Verification items for the finished model (mm, model axes). Round coordinates to 2 decimals unless told otherwise and drop trailing zeros. Write each loop counter-clockwise with the first axis right and the second up, starting at its lowest first coordinate (ties: lowest second). Pieces come first, ordered by that corner, then holes. Notation, with made-up numbers: (20, -34.75) - (54, -34.75) arc R19 ccw to (54, -5.75) - close; hole circle Ø5 at (-10, -2). An arc over 180 degrees is marked (long way). Answer as a JSON object with one key per item and string values.
```python
from build123d import *

# Parameters (mm, degrees)
SKETCH1_W           = 120
SKETCH1_H           = 50
BOSS_EXTRUDE1_DEPTH = 5
SKETCH4_R           = 17.4
CUT_EXTRUDE3_DEPTH  = 2
CUT_EXTRUDE2_DEPTH  = 5
BOSS_EXTRUDE2_DEPTH = 4
CIRPATTERN1_COUNT   = 4
SKETCH6_R           = 1.6
CUT_EXTRUDE4_DEPTH  = 131.096118313
SKETCH8_W           = 56
SKETCH8_H           = 28
CUT_EXTRUDE5_DEPTH  = 131.096118313
SKETCH9_W           = 44
SKETCH9_H           = 40
CUT_EXTRUDE6_DEPTH  = 3
SKETCH10_W          = 56
SKETCH10_H          = 40
CUT_EXTRUDE7_DEPTH  = 1
SKETCH11_R          = 1.6
CUT_EXTRUDE8_DEPTH  = 131.096118313
CHAMFER1_SIZE       = 1
CHAMFER2_SIZE       = 1


with BuildPart() as part:
    # Sketch1 → Boss-Extrude1 (new body)
    with BuildSketch(Plane(origin=(0, 0, 0), x_dir=(1, 0, 0), z_dir=(0, 1, 0))):
        with Locations((60, 25)):
            Rectangle(SKETCH1_W, SKETCH1_H)
    extrude(amount=BOSS_EXTRUDE1_DEPTH)

    # Sketch4 → Cut-Extrude3 (cut)
    with BuildSketch(Plane(origin=(0, 5, 0), x_dir=(1, 0, 0), z_dir=(0, 1, 0))):
        with Locations(Location((25, 25, 0), (0, 0, 270))):
            Circle(SKETCH4_R)
    extrude(amount=-CUT_EXTRUDE3_DEPTH, mode=Mode.SUBTRACT)

    # Sketch3 → Cut-Extrude2 (cut)
    with BuildSketch(Plane(origin=(0, 5, 0), x_dir=(1, 0, 0), z_dir=(0, 1, 0))):
        with BuildLine():
            Line((15, 36.5), (35, 36.5))
            ThreePointArc((35, 36.5), (36.414213562, 35.914213562), (37, 34.5))
            Line((37, 34.5), (37, 15.5))
            ThreePointArc((37, 15.5), (36.414213562, 14.085786438), (35, 13.5))
            Line((35, 13.5), (15, 13.5))
            ThreePointArc((15, 13.5), (13.585786438, 14.085786438), (13, 15.5))
            Line((13, 15.5), (13, 34.5))
            ThreePointArc((13, 34.5), (13.585786438, 35.914213562), (15, 36.5))
        make_face()
    extrude(amount=-CUT_EXTRUDE2_DEPTH, mode=Mode.SUBTRACT)

    # Sketch5 → Boss-Extrude2 (add)
    with BuildSketch(Plane(origin=(0, 3, 0), x_dir=(1, 0, 0), z_dir=(0, 1, 0))):
        with BuildLine():
            Line((9.8, 28.75), (11, 28.75))
            ThreePointArc((11, 28.75), (11.282842712, 28.632842712), (11.4, 28.35))
            Line((11.4, 28.35), (11.4, 21.65))
            ThreePointArc((11.4, 21.65), (11.282842712, 21.367157288), (11, 21.25))
            Line((11, 21.25), (9.8, 21.25))
            ThreePointArc((9.8, 21.25), (9.517157288, 21.367157288), (9.4, 21.65))
            Line((9.4, 21.65), (9.4, 28.35))
            ThreePointArc((9.4, 28.35), (9.517157288, 28.632842712), (9.8, 28.75))
        make_face()
    boss_extrude2 = extrude(amount=BOSS_EXTRUDE2_DEPTH)

    # CirPattern1: Boss-Extrude2 ×4 about axis
    cirpattern1_axis = Axis((25, 0, -25), (0, 1, 0))
    for i in range(1, CIRPATTERN1_COUNT):
        add(boss_extrude2.rotate(cirpattern1_axis, i * 360 / CIRPATTERN1_COUNT))

    # Sketch6 → Cut-Extrude4 (cut, through all)
    with BuildSketch(Plane(origin=(0, 5, 0), x_dir=(1, 0, 0), z_dir=(0, 1, 0))):
        with Locations(Location((4, 46, 0), (0, 0, 270))):
            Circle(SKETCH6_R)
        with Locations(Location((116, 46, 0), (0, 0, 270))):
            Circle(SKETCH6_R)
        with Locations(Location((116, 4, 0), (0, 0, 270))):
            Circle(SKETCH6_R)
        with Locations(Location((4, 4, 0), (0, 0, 270))):
            Circle(SKETCH6_R)
    extrude(amount=-CUT_EXTRUDE4_DEPTH, mode=Mode.SUBTRACT)

    # Sketch8 → Cut-Extrude5 (cut, through all)
    with BuildSketch(Plane(origin=(0, 5, 0), x_dir=(1, 0, 0), z_dir=(0, 1, 0))):
        with Locations((78, 25)):
            Rectangle(SKETCH8_W, SKETCH8_H)
    extrude(amount=-CUT_EXTRUDE5_DEPTH, mode=Mode.SUBTRACT)

    # Sketch9 → Cut-Extrude6 (cut)
    with BuildSketch(Plane(origin=(0, 0, 0), x_dir=(1, 0, 0), z_dir=(0, 1, 0))):
        with Locations((78, 25)):
            Rectangle(SKETCH9_W, SKETCH9_H)
    extrude(amount=CUT_EXTRUDE6_DEPTH, mode=Mode.SUBTRACT)

    # Sketch10 → Cut-Extrude7 (cut)
    with BuildSketch(Plane.XZ):
        with Locations((78, -25)):
            Rectangle(SKETCH10_W, SKETCH10_H)
    extrude(amount=-CUT_EXTRUDE7_DEPTH, mode=Mode.SUBTRACT)

    # Sketch11 → Cut-Extrude8 (cut, through all)
    with BuildSketch(Plane(origin=(0, 5, 0), x_dir=(1, 0, 0), z_dir=(0, 1, 0))):
        with Locations(Location((52.9, 41.8, 0), (0, 0, 270))):
            Circle(SKETCH11_R)
        with Locations(Location((103.099401804, 42.045068405, 0), (0, 0, 270))):
            Circle(SKETCH11_R)
        with Locations(Location((103.099812841, 8.445068408, 0), (0, 0, 270))):
            Circle(SKETCH11_R)
        with Locations(Location((52.9, 8.445068408, 0), (0, 0, 270))):
            Circle(SKETCH11_R)
    extrude(amount=-CUT_EXTRUDE8_DEPTH, mode=Mode.SUBTRACT)

    # Chamfer1
    chamfer1_edges = [part.edges().sort_by_distance(p)[0] for p in [
        (120, 5, -25),
        (60, 5, -50),
        (0, 5, -25),
        (60, 0, -50),
        (120, 0, -25),
        (60, 0, 0),
        (0, 0, -25),
        (0, 2.5, -50),
        (120, 2.5, -50),
        (120, 2.5, 0),
        (0, 2.5, 0),
        (60, 5, 0),
    ]]
    chamfer(chamfer1_edges, length=CHAMFER1_SIZE)

    # Chamfer2
    # the kernel refuses this chamfer: 1 mm, written as the material it takes off along each edge
    with BuildSketch(Plane(origin=(106, 5, -11), x_dir=(0, 0.02749587661058651, 0.9996219169112968), z_dir=(-1, 0, 0)), Plane(origin=(50, 5, -39), x_dir=(0, 0.027495876610586414, -0.9996219169112968), z_dir=(1, 0, 0))) as chamfer2_piece_1:
        Polygon((CHAMFER2_SIZE * 0.999621916911, -CHAMFER2_SIZE * 0.0274958766106), (-CHAMFER2_SIZE * 0.0274958766106, -CHAMFER2_SIZE * 0.999621916911), (0, 0), align=None)
    extrude(amount=56, mode=Mode.SUBTRACT)


solid = part.part
```
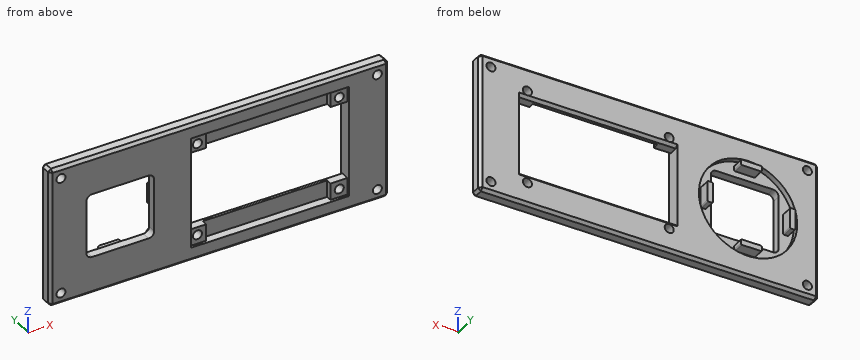
Q1. Section check C-C, the plane x = 116. Record the cut outline in (y, z).
Geometry check:
{"outline": "(0, -49) - (1, -50) - (4, -50) - (5, -49) - (5, -47.6) - (0, -47.6) - close; (0, -44.4) - (5, -44.4) - (5, -5.6) - (0, -5.6) - close; (0, -2.4) - (5, -2.4) - (5, -1) - (4, 0) - (1, 0) - (0, -1) - close"}
Q2. Section check A-A, the plane x = 25. Record the cut outline in (y, z), then the cut area to 3 significant figures.
Geometry check:
{"outline": "(0, -49) - (1, -50) - (4, -50) - (5, -49) - (5, -42.4) - (3, -42.4) - (3, -40.6) - (7, -40.6) - (7, -38.6) - (3, -38.6) - (3, -36.5) - (0, -36.5) - close; (0, -13.5) - (3, -13.5) - (3, -11.4) - (7, -11.4) - (7, -9.4) - (3, -9.4) - (3, -7.6) - (5, -7.6) - (5, -1) - (4, 0) - (1, 0) - (0, -1) - close", "area": "125 mm2"}
Q3. Section check B-B, the plane z = -25. Record the cut outline in (x, y).
Geometry check:
{"outline": "(0, 1) - (1, 0) - (13, 0) - (13, 3) - (11.4, 3) - (11.4, 7) - (9.4, 7) - (9.4, 3) - (7.6, 3) - (7.6, 5) - (1, 5) - (0, 4) - close; (37, 0) - (50, 0) - (50, 5) - (42.4, 5) - (42.4, 3) - (40.6, 3) - (40.6, 7) - (38.6, 7) - (38.6, 3) - (37, 3) - close; (106, 0) - (119, 0) - (120, 1) - (120, 4) - (119, 5) - (106, 5) - close"}
Q4. Material ranges on line 1 along X through (y, z) = (3.85, -4); line 2 along X through (y, z) = (1.5, -8.5); line 3 along Z through (x, y) = (116, 1.4), recorded low to high. Write a range as [from, to].
Geometry check:
{"line 1": "x = [0, 2.4], [5.6, 114.4], [117.6, 120]", "line 2": "x = [0, 51.3], [54.5, 56], [100, 101.5], [104.7, 120]", "line 3": "z = [-50, -47.6], [-44.4, -5.6], [-2.4, 0]"}
Q5. Section check D-D, the plane x = 48. Record the cut outline in (y, z), then the cut area to 3 significant figures.
Geometry check:
{"outline": "(0, -49) - (1, -50) - (4, -50) - (5, -49) - (5, -1) - (4, 0) - (1, 0) - (0, -1) - close", "area": "248 mm2"}
Q6. Gauge pin test, flat ends, axial feed: P1, Ø1.9, axis at x = 103.1, z = -42.05, coming from the -Y side; P2, Ø0.6, axis at x = 39.5, y = 5, coming from the -Z side; P3, Ø4, axis at x = 35.5, z = -30.5, coming from the +Y side; P4, Ø5, axis at x = 53.5, z = -9.5, coming from the -Y side. Record the tip position at first contact, or that the pin passes through.
Geometry check:
{"P1": "passes through", "P2": "stops at z = -49.3", "P3": "stops at y = 3", "P4": "stops at y = 1"}
